```python
from build123d import *

# Parameters (mm, degrees)
F2_R = 3


with BuildPart() as f1:
    # F0 (on Front) → F1 (revolve)
    with BuildSketch(Plane.XZ):
        Polygon((-27.94, 0), (0, 0), (0, 7), (-22, 7), (-22, 82.55), (-27.94, 82.55), align=None)
    revolve(axis=Axis((0, 0, 3.5), (0, 0, -1)))

    # F2
    f2_edges = [f1.edges().sort_by_distance(p)[0] for p in [
        (22, 0, 82.55),
        (27.94, 0, 0),
    ]]
    fillet(f2_edges, radius=F2_R)

    # F6: sweep along a path in F4
    with BuildLine(Plane.XZ) as f6_path:
        ThreePointArc((-27.9568824917, 75.0939920545), (-60.8796643301, 45.6174495611), (-28.1154159456, 15.9647911787))
    # F5 (on line) → F6 (sweep)
    with BuildSketch(Plane(origin=(-22, 0, 0), x_dir=(0, -1, 0), z_dir=(-1, 0, 0))):
        with BuildLine():
            add(Edge.make_bspline(
                [(8.2423, 75.3380134702), (8.2423, 84.1801954249), (-4.12115, 79.7591044475), (-16.4846, 75.3380134702), (-4.12115, 70.9169224928), (8.2423, 66.4958315155), (8.2423, 75.3380134702)],
                knots=[0, 0, 0, 2.0943951024, 2.0943951024, 4.1887902048, 4.1887902048, 6.2831853072, 6.2831853072, 6.2831853072], degree=2, weights=[1, 0.5, 1, 0.5, 1, 0.5, 1]))
        make_face()
    sweep(path=f6_path.line)


solid = f1.part
```
Read the model definition and answer for the solid it produces. Units are mm, in the model's axes. Give positions to 0.01 mm unless a question says otherwise; leave off trailing zeros. Order: outer loops, then holes, each group sorted by start corner. A loop starts at its lowest first (then second) coordinate and runs counter-clockwise, first axis right, second up. Notation, with made-up numbers: (35.25, 64) -> (64.25, 64) arc R20 ccw to (64.25, 100) -> close; hole circle Ø11 at (-38, -26). An arc over 180 degrees is marked (long way). One line per item, written item: value. Start each with the question number.
(1) The part is cut by section A-A (x = 0). Determine the outline of the cut face in (y, z), and give its area (3 significant figures).
(2) Flat-ended cylindrical pins translate along their axes: P1, Ø8, axis at x = -49, z = 72.5, coming from the -Y side; P2, Ø8, axis at x = 2, z = 43.5, coming from the -Y side; P3, Ø6, axis at x = -11.5, z = 50, coming from the -Y side; P4, Ø2, axis at x = -4, y = -13.5, coming from the -Z side. Find the tip coordinate at first contact, or state that the pin passes through.
(3) The part is cut by section B-B (z = 47). State how many separate pieces and enclosed holes the cut face has, and give its area (3 significant figures).
(4) Straight lines are drawn through the part: L1, parallel to X at y = 7, z = 37.5; L2, parallel to Y at x = 0, z = 47.5; L3, parallel to X at y = 2.5, z = 33. For each, find the intervals that lie inside material, in ascending order.
(5) For a pull along Z with two mould halves and no side action, classify faces 1 (the cylindrical face through (4.769, -21.477, 43.783)), 2 (the flat face through (-21, -14, 82.55)), 3 (the flat face through (-33.88, -0.52, 14.44)), 4 (the flat face through (0, 0, 0)) as released by +Z, released by -Z, zero draft, split by the parting line, or undercut.
Taken from the geometry:
1. outline: (-27.94, 3) arc R3 ccw to (-24.94, 0) -> (24.94, 0) arc R3 ccw to (27.94, 3) -> (27.94, 82.55) -> (25, 82.55) arc R3 ccw to (22, 79.55) -> (22, 7) -> (-22, 7) -> (-22, 79.55) arc R3 ccw to (-25, 82.55) -> (-27.94, 82.55) -> close
1. area: 1,280 mm^2
2. P1: y = -8.24
2. P2: y = -27.94
2. P3: y = -26.62
2. P4: z = 0
3. separate pieces: 2
3. enclosed holes: 1
3. area: 1,060 mm^2
4. L1: -63.94 to -58.61, -27.05 to -20.86, 20.86 to 27.05
4. L2: -27.94 to -22, 22 to 27.94
4. L3: -64.74 to -54.57, -27.83 to -21.86, 21.86 to 27.83
5. face 1: zero draft
5. face 2: released by +Z
5. face 3: undercut
5. face 4: released by -Z
